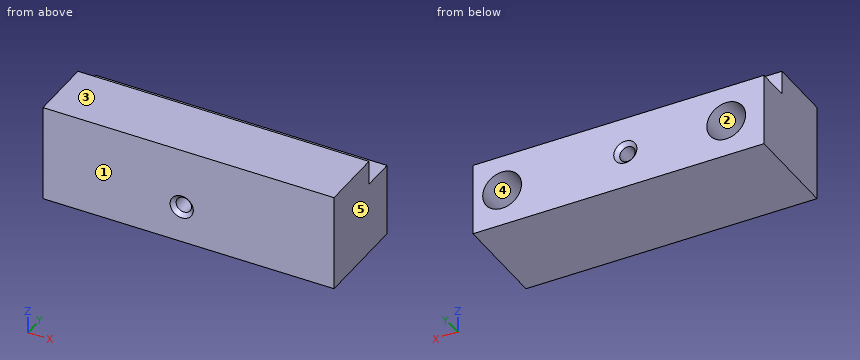
from build123d import *

# Parameters (mm, degrees)
BOSS_EXTRUDE1_DEPTH      = 38.1
BOSS_EXTRUDE1_DEPTH_BACK = 38.1
SKETCH2_R                = 5.08
CUT_EXTRUDE1_DEPTH       = 19.05
F_10_32_TAPPED_HOLE2_D   = 4.0386
CHAMFER5_SIZE            = 1.016
CHAMFER6_SIZE            = 1.016


with BuildPart() as part:
    # Sketch1 → Boss-Extrude1 (new body, two sides)
    with BuildSketch(Plane(origin=(0, 0, 0), x_dir=(0, 0, -1), z_dir=(1, 0, 0))) as boss_extrude1_sk:
        Polygon((0, 0), (-6.35, 0), (-6.35, -16.764), (19.05, -16.764), (19.05, 8.636), (0, 8.636), align=None)
    extrude(amount=BOSS_EXTRUDE1_DEPTH)
    extrude(boss_extrude1_sk.sketch, amount=-BOSS_EXTRUDE1_DEPTH_BACK)

    # Sketch2 → Cut-Extrude1 (cut)
    with BuildSketch(Plane(origin=(0, 8.636, 0), x_dir=(1, 0, 0), z_dir=(0, 1, 0))):
        with Locations((-28.194, 9.398)):
            Circle(SKETCH2_R)
        with Locations((30.48, 9.398)):
            Circle(SKETCH2_R)
    extrude(amount=-CUT_EXTRUDE1_DEPTH, mode=Mode.SUBTRACT)

    # 10-32 Tapped Hole2 (through all)
    with Locations(Plane(origin=(-1.778, 8.636, -9.398), x_dir=(0, 0, 1), z_dir=(0, 1, 0))):
        with Locations((0, 0)):
            Hole(F_10_32_TAPPED_HOLE2_D / 2)

    # Chamfer5
    chamfer5_edges = [part.edges().sort_by_distance(p)[0] for p in [
        (-1.778, 8.636, -7.3787),
    ]]
    chamfer(chamfer5_edges, length=CHAMFER5_SIZE)

    # Chamfer6
    chamfer6_edges = [part.edges().sort_by_distance(p)[0] for p in [
        (-1.778, -16.764, -7.3787),
    ]]
    chamfer(chamfer6_edges, length=CHAMFER6_SIZE)


solid = part.part
Design review of the part built by this model. Coordinates are the model's own, in mm. Face numbers are marked on the shaded views. A direction names the side the tool comes from. Round coordinates to 2 decimals unless told otherwise and drop trailing zeros. Write each loop counter-clockwise with the first axis right and the second up, starting at its lowest first coordinate (ties: lowest second). Pieces come first, ordered by that corner, then holes. Notation, with made-up numbers: M 55.5,50.5 L 68.5,50.5 A19 cw 68.5,64.5 Z; hole C -0.5,42.5 d11. An arc over 180 degrees is marked long. One line per item, written item: value. Start each with the question number.
1. Take a section at D-D on x = 15. State the section outline as (y, z) points.
2. Take a section at A-A on y = 4.25. State the section outline as (x, z) points, then the cut area to 3 significant figures.
3. For the marked faces 4 and 5, list the 3-axis set-ups (+Z, -Z, +X, -X, +Y, -Y) from which the entire face can be reached by the end or side of a thin tool; tool diameter is ignored.
4. Take a section at B-B on x = 30.48. State the section outline as (y, z) points.
5. To check wall thickness, follow probe 1 along Z at (x, y) = (19, 1.75); probe 2 along X at (y, z) = (-6.5, -12.5); probe 3 along Z at (x, y) = (30.48, 2.5). State the ranges of each line that lie inside material, in increasing order. Write a range as from..to.
6. Clearance check with flat-ended pins moving along their axes: P1, Ø3, axis at x = 32, z = -11.5, coming from the +Y side; P2, Ø4.5, axis at x = -1.778, z = -9.398, coming from the +Y side; P3, Ø7, axis at x = -16.5, y = 4.5, coming from the +Z side. State where each tip first meets the part, or that it passes through.
7. Take a section at C-C on y = -7.75. State the section outline as (x, z) points.
8. Draft analysis for pull direction Z (two halves, no side actions). For the marked faces 1, 2 and 3, state which applies: pulls with the +Z half, pulls with the -Z half, needs draft (parallel to the pull), parting line crosses it, or undercut.
Computed:
1. outline: M -16.76,-19.05 L 8.64,-19.05 L 8.64,0 L 0,0 L 0,6.35 L -16.76,6.35 Z
2. outline: M -38.1,-19.05 L 38.1,-19.05 L 38.1,0 L -38.1,0 Z; hole C -28.19,-9.4 d10.16; hole C -1.78,-9.4 d4.04; hole C 30.48,-9.4 d10.16
2. area: 1,280 mm²
3. face 4: +Y
3. face 5: +Z, -Z, +X, +Y, -Y
4. outline: M -16.76,-19.05 L 8.64,-19.05 L 8.64,-14.48 L -10.41,-14.48 L -10.41,-4.32 L 8.64,-4.32 L 8.64,0 L 0,0 L 0,6.35 L -16.76,6.35 Z
5. probe 1: z = -19.05..0
5. probe 2: x = -38.1..-32.22, -24.17..26.46, 34.5..38.1
5. probe 3: z = -19.05..-14.48, -4.32..0
6. P1: stops at y = -10.41
6. P2: stops at y = 7.85
6. P3: stops at z = 0
7. outline: M -38.1,-19.05 L 38.1,-19.05 L 38.1,6.35 L -38.1,6.35 Z; hole C -28.19,-9.4 d10.16; hole C -1.78,-9.4 d4.04; hole C 30.48,-9.4 d10.16
8. face 1: needs draft
8. face 2: undercut
8. face 3: pulls with the +Z half
